```python
from build123d import *

# Parameters (mm, degrees)
SKETCH1_W           = 11
SKETCH1_H           = 11
BOSS_EXTRUDE1_DEPTH = 3.7
FILLET1_R           = 1
SKETCH2_W           = 3.3
SKETCH2_H           = 3.3
CUT_EXTRUDE1_DEPTH  = 2.55
SKETCH3_R           = 1.5
CUT_EXTRUDE2_DEPTH  = 9.613361713


with BuildPart() as part:
    # Sketch1 → Boss-Extrude1 (new body)
    with BuildSketch(Plane(origin=(0, 0, 0), x_dir=(1, 0, 0), z_dir=(0, 1, 0))):
        Rectangle(SKETCH1_W, SKETCH1_H)
    extrude(amount=BOSS_EXTRUDE1_DEPTH)

    # Fillet1
    fillet1_edges = [part.edges().sort_by_distance(p)[0] for p in [
        (5.5, 1.85, 5.5),
        (-5.5, 1.85, 5.5),
        (-5.5, 1.85, -5.5),
        (5.5, 1.85, -5.5),
    ]]
    fillet(fillet1_edges, radius=FILLET1_R)

    # Sketch2 → Cut-Extrude1 (cut)
    with BuildSketch(Plane(origin=(0, 3.7, 0), x_dir=(1, 0, 0), z_dir=(0, 1, 0))):
        with Locations((-2.825, 0)):
            Rectangle(SKETCH2_W, SKETCH2_H)
        with Locations((2.825, 0)):
            Rectangle(SKETCH2_W, SKETCH2_H)
    extrude(amount=-CUT_EXTRUDE1_DEPTH, mode=Mode.SUBTRACT)

    # Sketch3 → Cut-Extrude2 (cut, through all)
    with BuildSketch(Plane(origin=(0, 3.7, 0), x_dir=(1, 0, 0), z_dir=(0, 1, 0))):
        with Locations(Location((-2.825, 0, 0), (0, 0, 270))):
            Circle(SKETCH3_R)
        with Locations(Location((2.825, 0, 0), (0, 0, 270))):
            Circle(SKETCH3_R)
    extrude(amount=-CUT_EXTRUDE2_DEPTH, mode=Mode.SUBTRACT)


solid = part.part
```
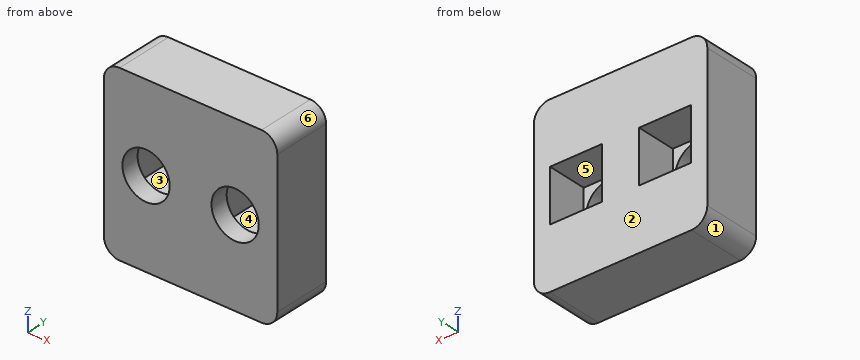
Work out the finished part from the listing and answer in its coordinate system (mm). Face numbers are marked on the shaded views. A direction names the side the tool comes from. Give positions to 0.01 mm unless a question says otherwise; leave off trailing zeros. Loops run counter-clockwise (first coordinate to the right, second up) from the corner with the lowest first, then second, coordinate; pieces in that order, holes last. Notation, with made-up numbers: (67, -8.75) - (75, -8.75) arc R32 cw to (75, 20.25) - close; hole circle Ø8 at (28.5, 56.25). An arc over 180 degrees is marked (long way). Use CSV: the item, a comma, the result in double quotes. Start each with the question number.
(1) Find the intervals of material crossed by L1, parallel to X at y = 0.5, z = 0 (3 decimals); L2, parallel to X at y = 2.95, z = -1 (3 decimals); L3, parallel to Z at x = 2.5, y = 1.65, in increasing order.
(2) Find section B-B, the plane z = 0. Determine the outline of the cut face in (x, y) (3 decimals).
(3) Find section C-C, the plane x = -4. Determine the outline of the cut face in (y, z), plus the area to 3 significant figures.
(4) A tool of negligible diameter and unlimited length cuts with its end or side. For the marked faces 5 and 6, from which of +Z, -Z, +X, -X, +Y, -Y can it reach the whole face along a straight path? Write none if from no direction.
(5) Determine the mould class of the marked faces 1, 2, 3 and 4 for opening direction Z: released by +Z, released by -Z, zero draft, split by the parting line, or undercut.
(6) Find section A-A, the plane y = 3.35. Determine the outline of the cut face in (x, z) (3 decimals).
(7) This flat-tipped pin is pushed along its axis until it touches: pin 1 (1.8 mm diameter, centred on x = -2.825, z = 0, fed in from -Y). Where does it stop, or does it pass through?
(8) Find section D-D, the plane x = -2.5. Determine the outline of the cut face in (y, z), plus the area to 3 significant figures.
Results found:
1,L1,"-5.5 to -4.325, -1.325 to 1.325, 4.325 to 5.5"
1,L2,"-5.5 to -4.475, -1.175 to 1.175, 4.475 to 5.5"
1,L3,"-5.5 to -1.65, 1.65 to 5.5"
2,outline,"(-5.5, 0) - (-4.325, 0) - (-4.325, 1.15) - (-4.475, 1.15) - (-4.475, 3.7) - (-5.5, 3.7) - close; (-1.325, 0) - (1.325, 0) - (1.325, 1.15) - (1.175, 1.15) - (1.175, 3.7) - (-1.175, 3.7) - (-1.175, 1.15) - (-1.325, 1.15) - close; (4.325, 0) - (5.5, 0) - (5.5, 3.7) - (4.475, 3.7) - (4.475, 1.15) - (4.325, 1.15) - close"
3,outline,"(0, -5.5) - (3.7, -5.5) - (3.7, -1.65) - (1.15, -1.65) - (1.15, -0.93) - (0, -0.93) - close; (0, 0.93) - (1.15, 0.93) - (1.15, 1.65) - (3.7, 1.65) - (3.7, 5.5) - (0, 5.5) - close"
3,area,"30.1 mm^2"
4,face 5,"+Y"
4,face 6,"+Z, +X, +Y, -Y"
5,face 1,"released by -Z"
5,face 2,"zero draft"
5,face 3,"undercut"
5,face 4,"undercut"
6,outline,"(-5.5, -4.5) arc R1 ccw to (-4.5, -5.5) - (4.5, -5.5) arc R1 ccw to (5.5, -4.5) - (5.5, 4.5) arc R1 ccw to (4.5, 5.5) - (-4.5, 5.5) arc R1 ccw to (-5.5, 4.5) - close; hole (-4.475, -1.65) - (-1.175, -1.65) - (-1.175, 1.65) - (-4.475, 1.65) - close; hole (1.175, -1.65) - (4.475, -1.65) - (4.475, 1.65) - (1.175, 1.65) - close"
7,pin 1,"through"
8,outline,"(0, -5.5) - (3.7, -5.5) - (3.7, -1.65) - (1.15, -1.65) - (1.15, -1.46) - (0, -1.46) - close; (0, 1.46) - (1.15, 1.46) - (1.15, 1.65) - (3.7, 1.65) - (3.7, 5.5) - (0, 5.5) - close"
8,area,"28.9 mm^2"
